Autodesk Fusion 360 part; units mm, degrees
sketch "Boceto5" plane through (0, 0, 0) normal (0, 1, 0) x (1, 0, 0)
  circle A0 centre (0, 0) radius 12
  circle A1 centre (0, 0) radius 20
  line L0 (0, -18) -> (0, 20) construction
  line L1 (0, 20) -> (22, 0) construction
  line L2 (22, 0) -> (-21, 0) construction
  circle A2 centre (0, -17) radius 2
  circle A3 centre (12.0208, -12.0208) radius 2
  circle A4 centre (17, 0) radius 2
  circle A5 centre (12.0208, 12.0208) radius 2
  circle A6 centre (0, 17) radius 2
  circle A7 centre (-12.0208, 12.0208) radius 2
  circle A8 centre (-17, 0) radius 2
  circle A9 centre (-12.0208, -12.0208) radius 2
  dimension "d1" = 24
  dimension "d2" = 40
  dimension "d3" = 8
  dimension "d4" = 4
  dimension "d5" = 17
  dimension "d7" = 360
extrude "Extruir1" add sketch "Boceto5" along normal blind 35
ref_plane "PlanoDeObra1" through (0, 27.7, 0) normal (0, 1, 0) x (1, 0, 0)
sketch "Boceto6" plane through (0, 27.7, 0) normal (0, 1, 0) x (1, 0, 0)
  circle A0 centre (0, 0) radius 13.2354
  circle A1 centre (0, 0) radius 5
  dimension "d11" = 10
extrude "Extruir2" add sketch "Boceto6" against normal blind 3
sketch "Boceto7" plane through (0, 0, 0) normal (0, -1, 0) x (1, 0, 0)
  circle A0 centre (-12.0208, 12.0208) radius 2
  circle A1 centre (12.0208, 12.0208) radius 2
  circle A2 centre (-12.0208, -12.0208) radius 2
  circle A3 centre (0, 0) radius 12
  circle A4 centre (17, 0) radius 2
  circle A5 centre (12.0208, -12.0208) radius 2
  circle A6 centre (-17, 0) radius 2
  circle A7 centre (0, -17) radius 2
  circle A8 centre (0, 17) radius 2
  circle A9 centre (0, 0) radius 20
  circle A10 centre (0, 0) radius 27
  circle A11 centre (0, 0) radius 12
extrude "Extruir3" add sketch "Boceto7" along normal blind 20 and the other way blind 4 contours A10
sketch "Boceto8" plane through (0, -20, 0) normal (0, -1, 0) x (1, 0, 0)
  circle A0 centre (0, 0) radius 20
  circle A1 centre (0, 0) radius 27
  spline S0 degree 5 poles (0.8049, -26.988) (-1.1916, -26.6528) (-5.0661, -25.9145) (-10.5223, -24.6033) (-17.129, -22.45) (-24.4438, -19.1245) (-30.9638, -15.2359) (-36.6141, -10.944) (-41.1579, -6.4179) (-43.6205, -2.0992) (-43.7018, 2.1218) (-41.8139, 6.6729) (-38.2196, 11.3661) (-32.8205, 15.2954) (-25.9465, 18.4821) (-17.9948, 21.1667) (-11.1308, 23.2874) (-5.8571, 25.0495) (-2.3066, 26.329) (-0.5226, 26.9949) knots 0 0 0 0 0 0 0.066667 0.133333 0.2 0.266667 0.333333 0.4 0.466667 0.533333 0.6 0.666667 0.733333 0.8 0.866667 0.933333 1 1 1 1 1 1
  spline S1 degree 5 poles (22.4701, -14.9698) (23.4209, -14.1205) (25.2562, -12.6285) (27.8097, -11.0079) (30.796, -9.7676) (33.7124, -8.1227) (35.6265, -5.0956) (36.3527, 0.0255) (35.6595, 4.9302) (33.5709, 7.4325) (30.4274, 8.6009) (27.3931, 9.8371) (24.9893, 11.8342) (23.3518, 13.7692) (22.5244, 14.888) knots 0 0 0 0 0 0 0.1 0.2 0.3 0.4 0.5 0.6 0.7 0.8 0.9 1 1 1 1 1 1
  line L0 (36, -3.7373) -> (36, 3.7373)
  line L1 (18.3284, -18.669) -> (26.6118, -11.2706)
  line L2 (26.1391, 10.0004) -> (18.9097, 19.7756)
  circle A2 centre (32, 0.1921) radius 2
  circle A3 centre (-31.1235, -10.1718) radius 2
  line L3 (-65, 0) -> (0, 0) construction
  line L4 (0, 0) -> (0, -32.1871) construction
  circle A4 centre (-31.1235, 10.1718) radius 2
  line L5 (-46.074, -0.0716) -> (-35.3734, 15.5371)
  circle A5 centre (0, 0) radius 27 construction
  line L6 (15.8053, -29.5065) -> (-14.1954, -24.4695)
  line L7 (-14.284, 21.8582) -> (13.2387, 32.1317)
  line L8 (-33.4619, -14.8868) -> (-46.5381, 0.3871)
  point P0 (-40, -7.2498)
  point P1 (-40.7237, 7.7327)
  point P2 (36, 0)
  dimension "d18" = 4
  dimension "d19" = 4
  dimension "d20" = 36
  dimension "d21" = 32
  dimension "d22" = 15
  dimension "d23" = 40
  dimension "d24" = 30
  dimension "d25" = 105
extrude "Extruir4" add sketch "Boceto8" against normal blind 6.5 contours A1 S1 | A1 S0 picked at (-33.9376, 4.4367)
ref_plane "PlanoDeObra2" through (-5, 0, 0) normal (1, 0, 0) x (0, 1, 0)
sketch "Boceto9" plane through (0, 0, 0) normal (0, -1, 0) x (1, 0, 0)
sketch "Boceto10" plane through (-5, 0, 0) normal (1, 0, 0) x (0, 1, 0)
  circle A0 centre (-19, 0) radius 4
  line L0 (-20, -23.6837) -> (-20, 21.762)
  dimension "d31" = 8
  dimension "d32" = 1
extrude "Extruir5" cut sketch "Boceto10" against normal blind 48
sketch "Boceto11" plane through (0, 4, 0) normal (0, 1, 0) x (-1, 0, 0)
  circle A0 centre (0, 0) radius 20
  circle A1 centre (0, 0) radius 27
Read the model definition and answer for the solid it produces. Units are mm, in the model's axes. A direction names the side the tool comes from. Give positions to 0.01 mm unless a question says otherwise; leave off trailing zeros. Write each loop counter-clockwise with the first axis right and the second up, starting at its lowest first coordinate (ties: lowest second). Pieces come first, ordered by that corner, then holes. Notation, with made-up numbers: M 45,77.5 L 90,77.5 A29 ccw 90,102.5 Z; hole C 23,81 d6. An arc over 180 degrees is marked long. One line per item, written item: value. Start each with the question number.
(1) Find section C-C (x = 17). Determine the outline of the cut face in (y, z), plus the area to 3 significant figures.
(2) Determine the mould class of faces 1 (the cylindrical face through (-1.08, 26.22, 4.88)), 2 (the cylindrical face through (24.94, -5.5, -10.34)), 3 (the flat face through (9, 35, 9)) for opening direction Z: pulls with the +Z half, pulls with the -Z half, needs draft (parallel to the pull), parting line crosses it, or undercut.
(3) Find section D-D (y = -1). Determine the outline of the cut face in (x, z).
(4) Find section A-A (x = 0). Give the number of separate pieces and of enclosed holes in the cut face, plus the area to 3 significant figures.
(5) Flat-ended cylindrical pins translate along their axes: pin 1 Ø2 at (y, z) = (4, -18.5) entering from +X; pin 2 Ø7 at (x, z) = (29.5, 3) entering from +Y; pin 3 Ø20 at (x, z) = (1.5, -9.5) entering from -Y. Find the tip coordinate at first contact, or state that the pin passes through.
(6) Find the intervals of material crossed by line 1 (X direction, y = 25.6, z = 0); line 2 (X direction, y = 11, z = 0); line 3 (X direction, y = -6.5, z = 0), in increasing order.
(7) A tool of negligible diameter and unlimited length cuts with its end or side. For faces 4 (the cylindrical face through (-18.6, 17.3, -1.2)), 5 (the cylindrical face through (-4.336, 19.283, -19.524)), 6 (the flat face through (5.2, 24.7, -0.2)), from which of +Z, -Z, +X, -X, +Y, -Y can it reach the whole face along a straight path? Write none if from no direction.
Results below:
1. outline: M -20,-20.98 L 4,-20.98 L 4,-10.54 L 35,-10.54 L 35,-2 L 0,-2 L 0,-10.54 L -20,-10.54 Z; M -20,10.54 L 0,10.54 L 0,2 L 35,2 L 35,10.54 L 4,10.54 L 4,20.98 L -20,20.98 Z
1. area: 1,100 mm^2
2. face 1: undercut
2. face 2: parting line crosses it
2. face 3: needs draft
3. outline: C 0,0 d54; hole C 0,0 d40
4. separate pieces: 4
4. enclosed holes: 0
4. area: 658 mm^2
5. pin 1: stops at x = 20.56
5. pin 2: stops at y = 4
5. pin 3: stops at y = 0
6. line 1: x = -20 to -19, -15 to -5, 5 to 15, 19 to 20
6. line 2: x = -20 to -19, -15 to -12, 12 to 15, 19 to 20
6. line 3: x = -27 to -20, 20 to 27
7. face 4: +Y, -Y
7. face 5: +Y
7. face 6: -Y
